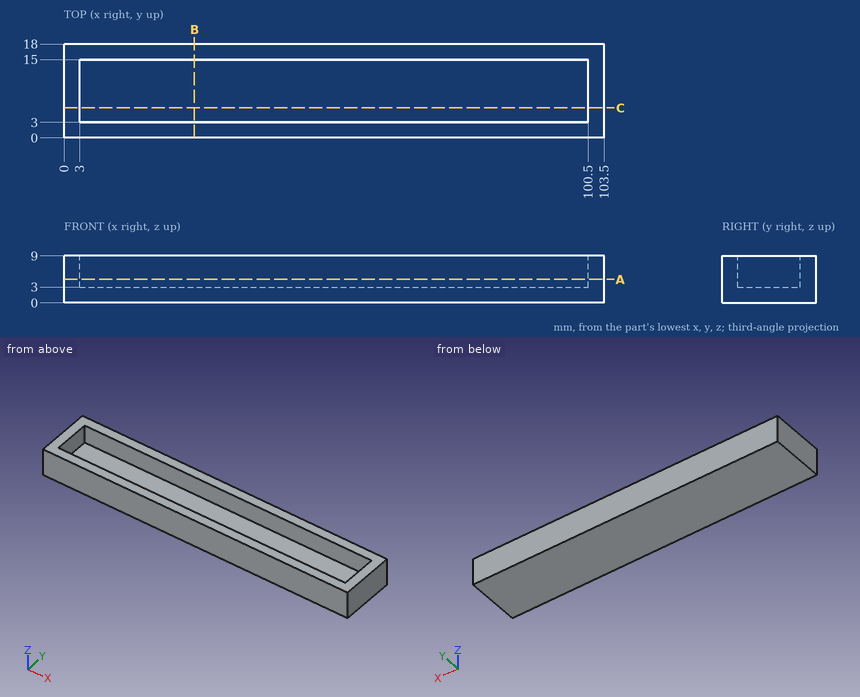
Drawing for the job (mm, zero at the part's lowest x, y, z). Coordinates: 2 decimals unless noted, no trailing zeros. Loops run counter-clockwise (first coordinate to the right, second up) from the corner with the lowest first, then second, coordinate; pieces in that order, holes last. Notation, with made-up numbers: (-3, 53) - (3, 53) arc R11 ccw to (3, 66) - close; hole circle Ø8 at (82, -21). An arc over 180 degrees is marked (long way). Use CSV: the item, a comma, the result in double quotes. Start each with the question number.
Q1. Cut at A-A, the plane z = 4.5. List the corners of the cut face in (x, y).
Q2. Cut at C-C, the plane y = 5.75. List the corners of the cut face in (x, z).
Q3. Drop a flat-ended pin along its axis: P1, Ø6, axis at x = 64.5, y = 6.5, coming from the +Z side. Give the stop position or say it passes through.
Q4. Probe probe 1 along Y at (x, z) = (28, 5.5); probe 2 along X at (y, z) = (4.75, 7.5); probe 3 along Z at (x, y) = (99, 14.5). List the from-to ranges inside material, lowest first. Write a range as from..to.
Q5. Cut at B-B, the plane x = 25. List the corners of the cut face in (y, z).
Here are the results:
1,outline,"(0, 0) - (103.5, 0) - (103.5, 18) - (0, 18) - close; hole (3, 3) - (100.5, 3) - (100.5, 15) - (3, 15) - close"
2,outline,"(0, 0) - (103.5, 0) - (103.5, 9) - (100.5, 9) - (100.5, 3) - (3, 3) - (3, 9) - (0, 9) - close"
3,P1,"z = 3"
4,probe 1,"0..3, 15..18"
4,probe 2,"0..3, 100.5..103.5"
4,probe 3,"0..3"
5,outline,"(0, 0) - (18, 0) - (18, 9) - (15, 9) - (15, 3) - (3, 3) - (3, 9) - (0, 9) - close"
